Work out the finished part from the listing and answer in its coordinate system (mm). A direction names the side the tool comes from. Coordinates: 2 decimals unless noted, no trailing zeros. Order: outer loops, then holes, each group sorted by start corner. A loop starts at its lowest first (then second) coordinate and runs counter-clockwise, first axis right, second up. Notation, with made-up numbers: M -1.5,-25 L 52.5,-25 A33 cw 52.5,10 Z; hole C -31.75,2 d6. An arc over 180 degrees is marked long. Use a Markdown table: item, result.
from build123d import *

# Parameters (mm, degrees)
SKETCH1_W                   = 7.8
SKETCH1_H                   = 17.45
SKETCH2_R                   = 2.5
CUT_EXTRUDE1_DEPTH          = 57.623758265
M6_TAPPED_HOLE2_D           = 5
M6_TAPPED_HOLE2_DEPTH       = 55
M6_TAPPED_HOLE2_CSINK_D     = 6.05
M6_TAPPED_HOLE2_CSINK_ANGLE = 90
M6_TAPPED_HOLE2_TIP         = 1.502151548
SKETCH5_R                   = 3
CUT_EXTRUDE2_DEPTH          = 56.966507842


with BuildPart() as part:
    # Sketch1 → Revolve1 (revolve)
    with BuildSketch(Plane.XY, mode=Mode.PRIVATE) as revolve1_sk:
        Polygon((28.1, 23.305), (1.6, 23.305), (0.065, 23.305), (1, 20.5), (1, 17.45), (0, 17.45), (0, 0), (28.7, 0), (28.7, 20.5), (29.7, 23.5), (29.7, 30), (28.1, 28.305), align=None)
        Polygon((0.065, 23.305), (1.6, 23.305), (1.6, 28.305), (0, 30), (0, 23.5), align=None)
        with Locations((-3.9, 8.725)):
            Rectangle(SKETCH1_W, SKETCH1_H)
    revolve(revolve1_sk.sketch.rotate(Axis((0, 0, 0), (1, 0, 0)), 90), axis=Axis((0, 0, 0), (1, 0, 0)))

    # Sketch2 → Cut-Extrude1 (cut, through all)
    with BuildSketch(Plane(origin=(29.7, 0, 0), x_dir=(0, 0, -1), z_dir=(1, 0, 0))):
        with Locations((12.5, 0)):
            Circle(SKETCH2_R)
        with Locations((0, -12.5)):
            Circle(SKETCH2_R)
        with Locations((-12.5, 0)):
            Circle(SKETCH2_R)
        with Locations((0, 12.5)):
            Circle(SKETCH2_R)
    extrude(amount=-CUT_EXTRUDE1_DEPTH, mode=Mode.SUBTRACT)

    # M6 Tapped Hole2
    with Locations(Plane(origin=(-7.8, 0, -12.5), x_dir=(0, 0, -1), z_dir=(-1, 0, 0))):
        with Locations((0, 0), (-12.5, -12.5), (-25, 0), (-12.5, 12.5)):
            CounterSinkHole(M6_TAPPED_HOLE2_D / 2, M6_TAPPED_HOLE2_CSINK_D / 2, depth=M6_TAPPED_HOLE2_DEPTH, counter_sink_angle=M6_TAPPED_HOLE2_CSINK_ANGLE)
            with Locations((0, 0, -(M6_TAPPED_HOLE2_DEPTH + M6_TAPPED_HOLE2_TIP / 2))):  # 118° drill point
                Cone(0, M6_TAPPED_HOLE2_D / 2, M6_TAPPED_HOLE2_TIP, mode=Mode.SUBTRACT)

    # Sketch5 → Cut-Extrude2 (cut, through all)
    with BuildSketch(Plane(origin=(28.7, 0, 0), x_dir=(0, 0, -1), z_dir=(1, 0, 0))):
        Circle(SKETCH5_R)
    extrude(amount=-CUT_EXTRUDE2_DEPTH, mode=Mode.SUBTRACT)


solid = part.part
(1) A cutting plane is placed at B-B (z = 0.5). Give the number of separate pieces and of enclosed holes in the cut face, then the cut area to 3 significant figures.
Conclusion:
| item | result |
|---|---|
| separate pieces | 4 |
| enclosed holes | 0 |
| area | 1,070 mm2 |
(2) Determine the mould class of faces 6 (the flat face through (-7.8, 0, -4)), 7 (the cylindrical face through (14.665, 14.181, -18.494)), 8 (the cylindrical face through (10.964, 0.751, 10.115)) for opening direction X: pulls with the +X half, pulls with the -X half, needs draft (parallel to the pull), parting line crosses it, or undercut.
Conclusion:
| item | result |
|---|---|
| face 6 | pulls with the -X half |
| face 7 | undercut |
| face 8 | needs draft |
(3) A cutting plane is placed at A-A (x = 19). Determine the outline of the cut face in (y, z) (3 decimals), then the cut area to 3 significant figures.
Conclusion:
| item | result |
|---|---|
| outline | C 0,0 d46.61; hole C -12.5,0 d5; hole C 0,0 d6; hole C 0,-12.5 d5; hole C 0,12.5 d5; hole C 12.5,0 d5 |
| area | 1,600 mm2 |
(4) Which of the six approach directions +Z, -Z, +X, -X, +Y, -Y give full straight-line access (tool end or side, diameter ignored) to faces 1 (the cylindrical face through (-3.462, 17.035, -3.783)), 2 (the flat face through (29.7, 20, -13)), 3 (the cylindrical face through (10.964, 0.751, -14.885)), 4 (the flat face through (28.7, 0, -4)), 5 (the flat face through (28.1, -23.2, 4.1))?
Conclusion:
| item | result |
|---|---|
| face 1 | -X |
| face 2 | +Z, -Z, +X, +Y, -Y |
| face 3 | +X, -X |
| face 4 | +X |
| face 5 | none |
(5) Given P1, Ø3, axis at y = 17.5, z = 6, coming from the +X side; P2, Ø4, axis at x = 6, z = -22.5, coming from the -Y side; P3, Ø8, axis at x = 21.5, z = -18.5, coming from the +Y side; P4, Ø3.5, axis at y = 0, z = 0, coming from the -X side, each flat-ended and moving along its own axis, determine where each tip first touches the part or whether it passes through.
Conclusion:
| item | result |
|---|---|
| P1 | x = 28.7 |
| P2 | y = -11.08 |
| P3 | y = 18.24 |
| P4 | through |
(6) Straight lines are drawn through the part: L1, parallel to Y at x = 19, z = 0 (3 decimals); L2, parallel to X at y = -5, z = 11.5; L3, parallel to Z at x = 3.5, y = -12.5. For each, find the intervals that lie inside material, in ascending order.
Conclusion:
| item | result |
|---|---|
| L1 | -23.305 to -15, -10 to -3, 3 to 10, 15 to 23.305 |
| L2 | -7.8 to 28.7 |
| L3 | -19.67 to -2.5, 2.5 to 19.67 |
